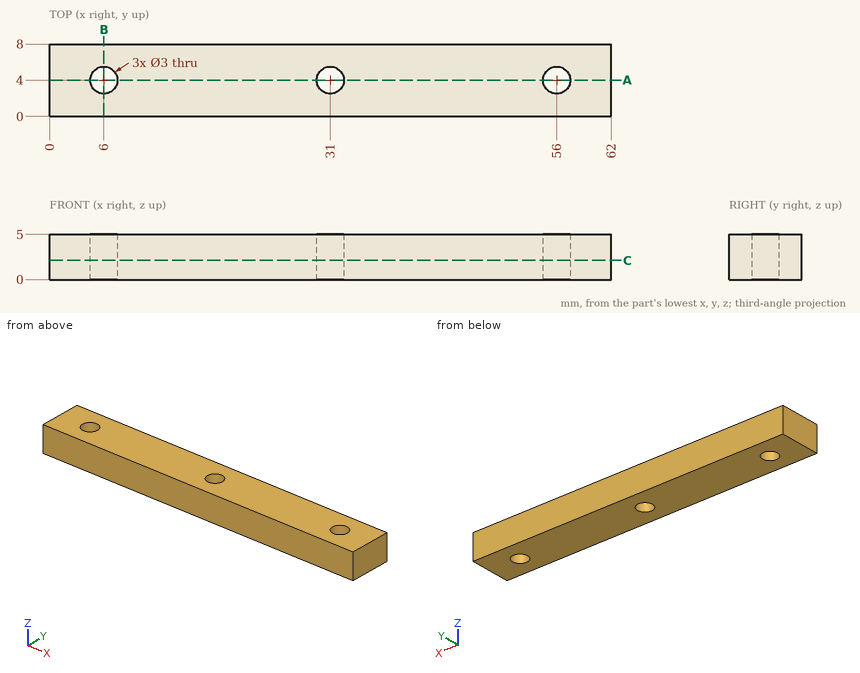
Check sheet for the drawn part. Datum: minimum x, y, z corner. Units: mm. Give positions to 0.01 mm unless a question says otherwise; leave off trailing zeros. Order: outer loops, then holes, each group sorted by start corner. A loop starts at its lowest first (then second) coordinate and runs counter-clockwise, first axis right, second up.
1. Scan lines: line 1 (Y direction, x = 56, z = 3.7); line 2 (X direction, y = 4.5, z = 1.3); line 3 (X direction, y = 4.75, z = 0.3). Record each from-to range of solid material in increasing order.
Completed:
line 1: y = 0 to 2.5, 5.5 to 8
line 2: x = 0 to 4.59, 7.41 to 29.59, 32.41 to 54.59, 57.41 to 62
line 3: x = 0 to 4.7, 7.3 to 29.7, 32.3 to 54.7, 57.3 to 62
2. Sectioned sample at A-A (y = 4). Record the boundary of the cut face in (x, z).
Completed:
outline: (0, 0) - (4.5, 0) - (4.5, 5) - (0, 5) - close; (7.5, 0) - (29.5, 0) - (29.5, 5) - (7.5, 5) - close; (32.5, 0) - (54.5, 0) - (54.5, 5) - (32.5, 5) - close; (57.5, 0) - (62, 0) - (62, 5) - (57.5, 5) - close
3. Sectioned sample at B-B (x = 6). Record the boundary of the cut face in (y, z).
Completed:
outline: (0, 0) - (2.5, 0) - (2.5, 5) - (0, 5) - close; (5.5, 0) - (8, 0) - (8, 5) - (5.5, 5) - close
4. Sectioned sample at C-C (z = 2.15). Record the boundary of the cut face in (x, y).
Completed:
outline: (0, 0) - (62, 0) - (62, 8) - (0, 8) - close; hole circle Ø3 at (6, 4); hole circle Ø3 at (31, 4); hole circle Ø3 at (56, 4)
5. Depth check by flat-ended pin: pin 1 (2.5 mm diameter, centred on x = 31, y = 4, fed in from +Z). Enter the tip coordinate at first touch or a pass-through.
Completed:
pin 1: passes through
